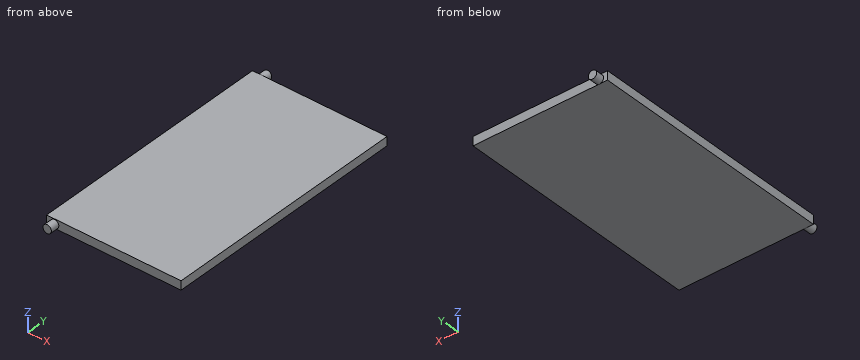
```python
from build123d import *

# Parameters (mm, degrees)
BOX_W             = 50
BOX_H             = 91.6
BOX_DEPTH         = 3.3
CYLINDER_R        = 1.56
CYLINDER_DEPTH    = 3.3
CYLINDER001_R     = 1.56
CYLINDER001_DEPTH = 3.3


with BuildPart() as part:
    # Box → Box (join)
    with BuildSketch(Plane.XY):
        with Locations((25, 45.8)):
            Rectangle(BOX_W, BOX_H)
    extrude(amount=BOX_DEPTH)

    # Cylinder → Cylinder (join)
    with BuildSketch(Plane(origin=(3, 0, 1.55), x_dir=(1, 0, 0), z_dir=(0, -1, 0))):
        Circle(CYLINDER_R)
    extrude(amount=CYLINDER_DEPTH)

    # Cylinder001 → Cylinder001 (join)
    with BuildSketch(Plane(origin=(3, 94.7, 1.55), x_dir=(1, 0, 0), z_dir=(0, -1, 0))):
        Circle(CYLINDER001_R)
    extrude(amount=CYLINDER001_DEPTH)


solid = part.part
```
Verification items for the finished model (mm, model axes). Give positions to 0.01 mm unless a question says otherwise; leave off trailing zeros. Loops run counter-clockwise (first coordinate to the right, second up) from the corner with the lowest first, then second, coordinate; pieces in that order, holes last. Notation, with made-up numbers: M 45,82 L 103,82 A17 ccw 103,114 Z; hole C -24.5,-14.5 d1. An arc over 180 degrees is marked long. One line per question, with ' | ' between items.
Item 1: Depth check by flat-ended pin: P1, Ø6, axis at x = 36, y = 80, coming from the -Z side; P2, Ø1.6, axis at x = 13, z = 2, coming from the +Y side; P3, Ø1.6, axis at x = 31.5, z = 2, coming from the -Y side. Enter the tip coordinate at first touch or a pass-through.
Completed:
P1: stops at z = 0 | P2: stops at y = 91.6 | P3: stops at y = 0
Item 2: Section check B-B, the plane x = 28. Record the cut outline in (y, z).
Completed:
outline: M 0,0 L 91.6,0 L 91.6,3.3 L 0,3.3 Z
Item 3: Section check A-A, the plane z = 1.55. Record the cut outline in (x, y).
Completed:
outline: M 0,0 L 1.44,0 L 1.44,-3.3 L 4.56,-3.3 L 4.56,0 L 50,0 L 50,91.6 L 4.56,91.6 L 4.56,94.7 L 1.44,94.7 L 1.44,91.6 L 0,91.6 Z
Item 4: Thickness scan on line 1 (Z direction, x = 3.5, y = 86.5); line 2 (Y direction, x = 16, z = 1.7). Record the ranges inside material, lowest first. Write a range as [from, to].
Completed:
line 1: z = [0, 3.3] | line 2: y = [0, 91.6]
